The model under review builds one solid part; all positions refer to its coordinate system, in mm. A direction names the side the tool comes from. Round coordinates to 2 decimals unless told otherwise and drop trailing zeros. Order: outer loops, then holes, each group sorted by start corner. A loop starts at its lowest first (then second) coordinate and runs counter-clockwise, first axis right, second up. Notation, with made-up numbers: M 34.5,78.5 L 91.5,78.5 A14 cw 91.5,97.5 Z; hole C -2.5,79 d2. An arc over 180 degrees is marked long. Answer as a JSON object with one key per item and string values. Group by question number.
1. Mouldability with a two-part tool opening along Z and no side actions: class faces 1 (the face through (-38.244, -101.021, -16.564)), 2 (the face through (-33, -27, 0)), 3 (the face through (-45.905, -35, -13)) as released by +Z, released by -Z, zero draft, split by the parting line, or undercut.
2. Machinability: for faces 4 (the face through (-33, -88.143, -13)), 5 (the face through (-28.81, 33.58, -12.52)), which of the approach directions +Z, -Z, +X, -X, +Y, -Y give a long, thin tool a straight path to every point of the face, cutting with its end or side? Answer none if there is none.
3. Clearance check with flat-ended pins moving along their axes: P1, Ø10, axis at x = -39.5, z = -17.5, coming from the +Y side; P2, Ø8, axis at x = -40, y = -95.5, coming from the +Z side; P3, Ø4, axis at x = -29.5, z = -14.5, coming from the -Y side; P4, Ø3, axis at x = -42, z = -18, coming from the +Y side. State where each tip first meets the part, or that it passes through.
4. Add section A-A on x = -38. State the section outline as (y, z) points.
5. To check wall thickness, follow probe 1 along Y at (x, z) = (-33, -19.5); probe 2 along Y at (x, z) = (-33, -12.75); probe 3 along Y at (x, z) = (-22.5, -13.75). State the ranges of each line that lie inside material, in increasing order. Write a range as [from, to].
```python
from build123d import *

# Parameters (mm, degrees)
F0_W     = 25.4
F0_H     = 171.45
F0_R     = 9.525
F1_DEPTH = 25.4
F2_R     = 12.69999
F3_R     = 6.35
F4_DEPTH = 25.4


# Not quite as in the source:
# - a fillet or chamfer is up to 0.001 mm smaller than in the source, because OpenCascade refuses the exact size


with BuildPart() as f1:
    # F0 (on Top) → F1 (new body)
    with BuildSketch(Plane.XY):
        with Locations((-33.2050182253, -27.8180489531)):
            Rectangle(F0_W, F0_H)
        with Locations((-33.2050182253, 42.0319510469)):
            Circle(F0_R, mode=Mode.SUBTRACT)
    extrude(amount=-F1_DEPTH)

    # F2 (radius 12.7 in the source; OpenCascade refuses exactly that, so slightly less here)
    f2_edges = [f1.edges().sort_by_distance(p)[0] for p in [
        (-45.905018, 57.906951, -12.7),
        (-20.505018, 57.906951, -12.7),
    ]]
    fillet(f2_edges, radius=F2_R)

    # F3 (on face) → F4 (cut)
    with BuildSketch(Plane.XZ.offset(113.5430489531)):
        with Locations((-33.2050182253, -12.7)):
            Circle(F3_R)
    extrude(amount=-F4_DEPTH, mode=Mode.SUBTRACT)


solid = f1.part
```
Recorded:
{
 "1": {"face 1": "undercut", "face 2": "released by +Z", "face 3": "zero draft"},
 "2": {"face 4": "-Y", "face 5": "+Z, -Z"},
 "3": {"P1": "stops at y = 57.84", "P2": "stops at z = 0", "P3": "stops at y = -88.14", "P4": "stops at y = 55.6"},
 "4": {"outline": "M -113.54,-25.4 L 33.8,-25.4 L 33.8,0 L -113.54,0 L -113.54,-8.54 L -88.14,-8.54 L -88.14,-16.86 L -113.54,-16.86 Z; M 50.26,-25.4 L 56.97,-25.4 L 56.97,0 L 50.26,0 Z"},
 "5": {"probe 1": "y = [-113.54, 32.51], [51.55, 57.91]", "probe 2": "y = [-88.14, 32.51], [51.55, 57.91]", "probe 3": "y = [-113.54, 52.04]"}
}
